Input: dimensioned drawing with shaded views. Units: mm. Origin: part minimum x, y, z. A direction names the side the tool comes from. Coordinates: 2 decimals unless noted, no trailing zeros. Order: outer loops, then holes, each group sorted by start corner. A loop starts at its lowest first (then second) coordinate and runs counter-clockwise, first axis right, second up. Notation, with made-up numbers: (29.25, 79) - (47.25, 79) arc R23 ccw to (47.25, 108) - close; hole circle Ø11 at (15, 32). An arc over 180 degrees is marked (long way). One line per question, with ' | ' between items. Start each with the question number.
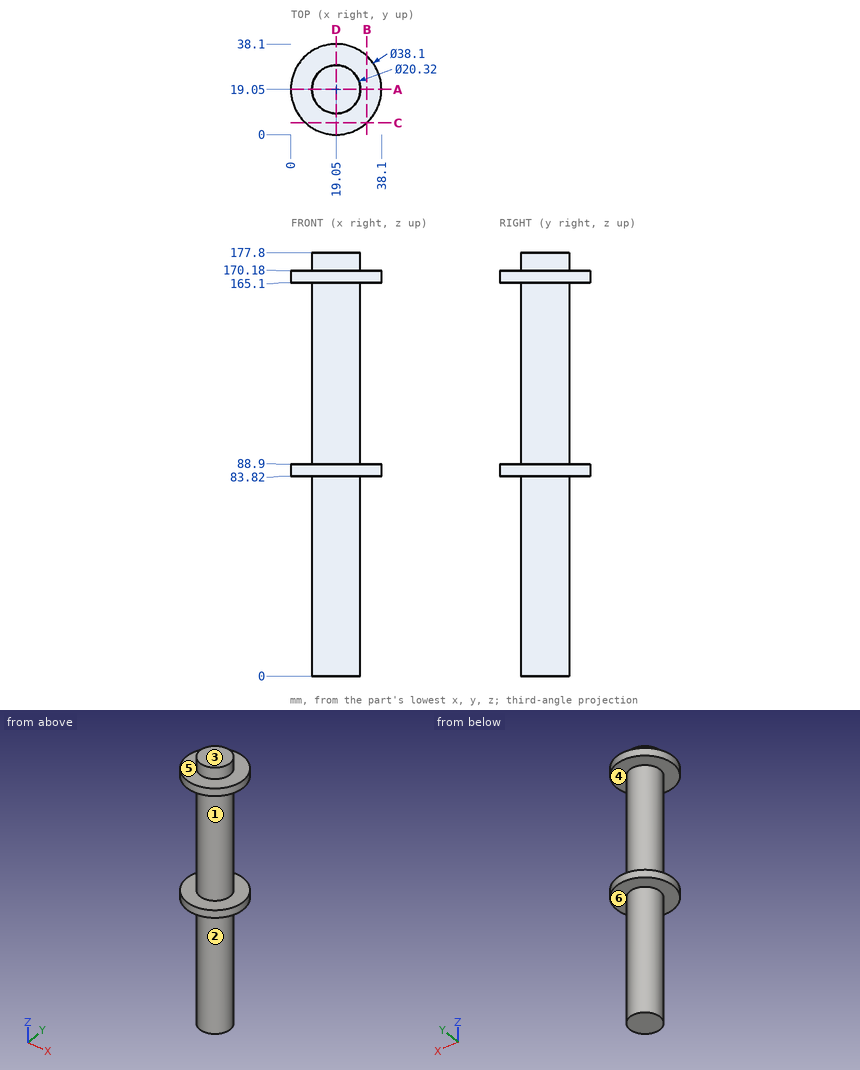
(1) Section A-A (y = 19.05). Output: boundary loops of the cut face in (x, z).
(2) Draft query along Z for the marked faces 4, 5 and 6. Return one class per face: +Z half, -Z half, draft (parallel to the pull), parting line (faces both ways), or undercut.
(3) Section B-B (x = 32). Output: boundary loops of the cut face in (y, z).
(4) Reachability of the marked faces 1, 2 and 3 from +Z, -Z, +X, -X, +Y, -Y: full face, straight path, thin tool, end or side. Return the list, or none.
(5) Material intervals for line 1 along Z through (x, y) = (13.5, 3); line 2 along X through (y, z) = (11, 51); line 3 along X through (y, z) = (12, 125), sorted ascending. Write a range as from..to.
(6) Section C-C (y = 5). Output: boundary loops of the cut face in (x, z).
(7) Pin query (flat end, axial travel): pin 1 (6 mm diameter, centred on y = 17, z = 34.5, fed in from +X); pin 2 (8 mm diameter, centred on y = 18, z = 44, fed in from -X); pin 3 (6 mm diameter, centred on x = 25.5, y = 5, fed in from +Z). Return the tip coordinate at first contact, or that it passes through.
Worked answers:
1) outline: (0, 83.82) - (8.89, 83.82) - (8.89, 0) - (29.21, 0) - (29.21, 83.82) - (38.1, 83.82) - (38.1, 88.9) - (29.21, 88.9) - (29.21, 165.1) - (38.1, 165.1) - (38.1, 170.18) - (29.21, 170.18) - (29.21, 177.8) - (8.89, 177.8) - (8.89, 170.18) - (0, 170.18) - (0, 165.1) - (8.89, 165.1) - (8.89, 88.9) - (0, 88.9) - close
2) face 4: undercut | face 5: +Z half | face 6: -Z half
3) outline: (5.08, 83.82) - (33.02, 83.82) - (33.02, 88.9) - (5.08, 88.9) - close; (5.08, 165.1) - (33.02, 165.1) - (33.02, 170.18) - (5.08, 170.18) - close
4) face 1: none | face 2: -Z | face 3: +Z, +X, -X, +Y, -Y
5) line 1: z = 83.82..88.9, 165.1..170.18 | line 2: x = 12.85..25.25 | line 3: x = 11.73..26.37
6) outline: (6.19, 83.82) - (31.91, 83.82) - (31.91, 88.9) - (6.19, 88.9) - close; (6.19, 165.1) - (31.91, 165.1) - (31.91, 170.18) - (6.19, 170.18) - close
7) pin 1: stops at x = 29.21 | pin 2: stops at x = 8.89 | pin 3: stops at z = 170.18
